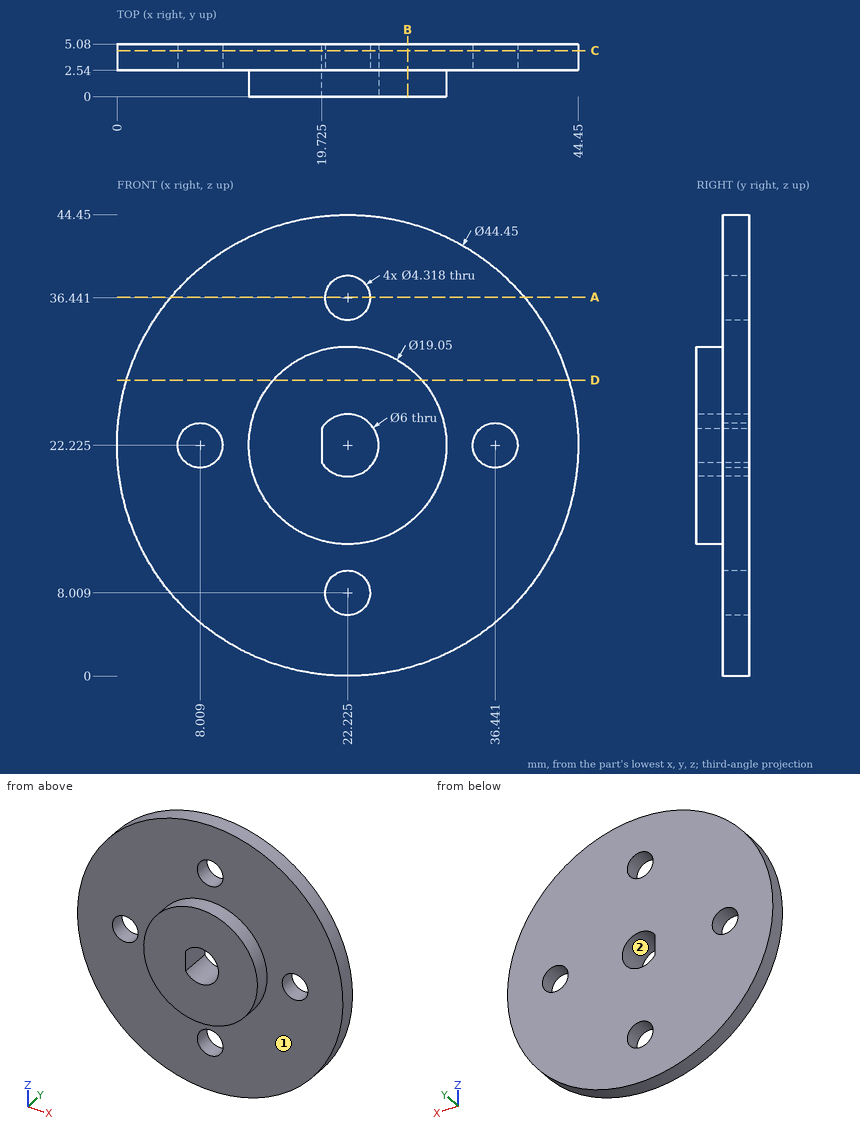
Design review of the part shown in the three views and the two pictorial views. Dimensions are in mm from the part's minimum x, y and z. Round coordinates to 2 decimals unless told otherwise and drop trailing zeros. Loops run counter-clockwise (first coordinate to the right, second up) from the corner with the lowest first, then second, coordinate; pieces in that order, holes last. Notation, with made-up numbers: (39, 58.25) -> (78, 58.25) arc R21 ccw to (78, 81.25) -> close; hole circle Ø10 at (35.25, -34). An arc over 180 degrees is marked (long way). Use one line per item in the form item = value. Start each with the question number.
Q1. Draft analysis for pull direction X (two halves, no side actions). For the marked faces 1 and 2, state which applies: +X half, -X half, draft (parallel to the pull), parting line (faces both ways), or undercut.
Q2. We need section A-A on z = 36.5. Give the boundary of the cut face in (x, y).
Q3. We need section D-D on z = 28.5. Give the boundary of the cut face in (x, y), then the cut area to 3 significant figures.
Q4. We need section C-C on y = 4.45. State how many separate pieces and enclosed holes the cut face has, then the cut area to 3 significant figures.
Q5. For pin 1 Ø7 at (x, z) = (8.01, 22.22) entering from -Y; pin 2 Ø8 at (x, z) = (13, 20) entering from -Y; pin 3 Ø3 at (y, z) = (1, 15) entering from -X; pin 4 Ø1.7 at (y, z) = (2, 23) entering from +X, all flat-tipped, find the tip position at first contact; note any pin that passes through.
Q6. Wall thickness on line 1 along X through (y, z) = (4.05, 22) (1 decimal); line 2 along Y through (x, z) = (13, 29); line 3 along Z through (x, y) = (24.5, 3.4) (1 decimal): over which ranges is each line inside the solid? List them lowest first. Write a range as [from, to].
Q7. We need section B-B on x = 28. Give the boundary of the cut face in (y, z).
Calculated:
q1.face_1 = draft
q1.face_2 = undercut
q2.outline = (5.19, 2.54) -> (20.07, 2.54) -> (20.07, 5.08) -> (5.19, 5.08) -> close; (24.38, 2.54) -> (39.26, 2.54) -> (39.26, 5.08) -> (24.38, 5.08) -> close
q3.outline = (0.9, 2.54) -> (15.06, 2.54) -> (15.06, 0) -> (29.39, 0) -> (29.39, 2.54) -> (43.55, 2.54) -> (43.55, 5.08) -> (0.9, 5.08) -> close
q3.area = 145 mm²
q4.separate_pieces = 1
q4.enclosed_holes = 5
q4.area = 1,470 mm²
q5.pin_1 = 2.54
q5.pin_2 = 0
q5.pin_3 = 14.61
q5.pin_4 = 44.45
q6.line_1 = [0, 5.9], [10.2, 19.7], [25.2, 34.3], [38.6, 44.4]
q6.line_2 = [2.54, 5.08]
q6.line_3 = [0.1, 20.3], [24.2, 44.3]
q7.outline = (0, 14.65) -> (2.54, 14.65) -> (2.54, 0.76) -> (5.08, 0.76) -> (5.08, 43.69) -> (2.54, 43.69) -> (2.54, 29.8) -> (0, 29.8) -> close
